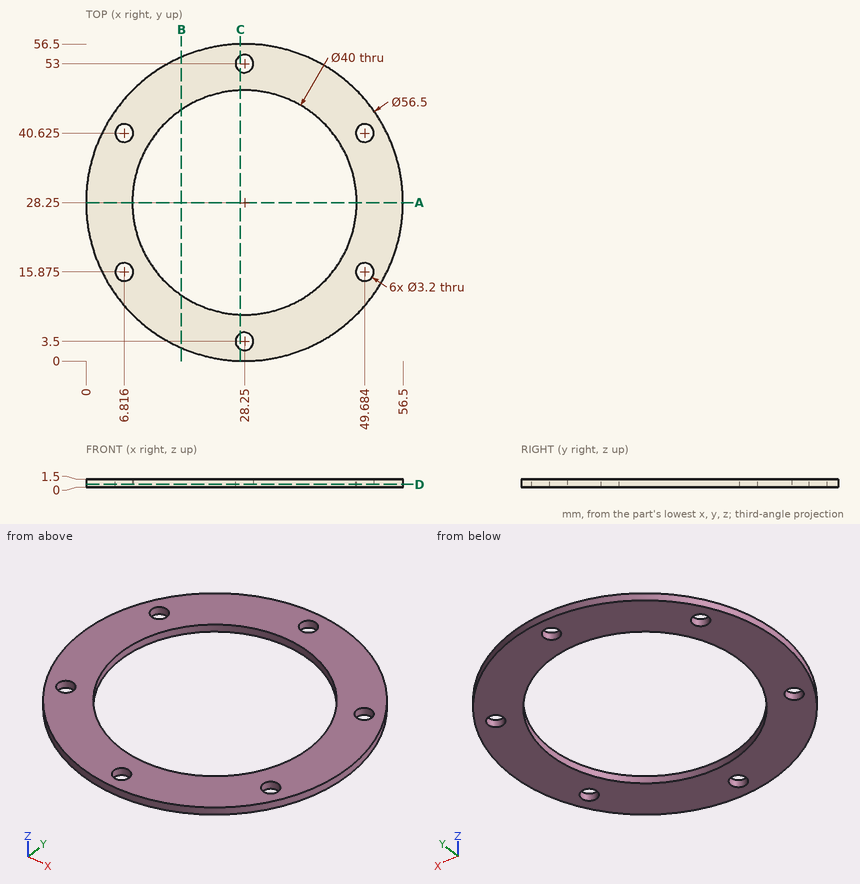
Job drawing, mm, ordinate dimensions from the low corner. One solid piece. Round coordinates to 2 decimals unless told otherwise and drop trailing zeros. Loops run counter-clockwise (first coordinate to the right, second up) from the corner with the lowest first, then second, coordinate; pieces in that order, holes last. Notation, with made-up numbers: (26, -6.75) -> (65, -6.75) arc R14 cw to (65, 12.25) -> close; hole circle Ø9 at (0, -4.5). An arc over 180 degrees is marked (long way). Use CSV: the item, a comma, the result in double quotes. Start each with the question number.
Q1. Saw through at C-C on x = 27.5. Give the cut face in (y, z).
Q2. Saw through at B-B on x = 17. Give the cut face in (y, z).
Q3. Drill centre lines: L1, parallel to Y at x = 28.25, z = 1.05; L2, parallel to X at y = 41, z = 0.45; L3, parallel to X at y = 17, z = 1. Where is each one in solid material? Low to high.
Q4. Saw through at A-A on y = 28.25. Give the cut face in (x, z).
Q5. Saw through at D-D on z = 0.55. Give the cut face in (x, y) (3 decimals).
Solutions:
1,outline,"(0.01, 0) -> (2.09, 0) -> (2.09, 1.5) -> (0.01, 1.5) -> close; (4.91, 0) -> (8.26, 0) -> (8.26, 1.5) -> (4.91, 1.5) -> close; (48.24, 0) -> (51.59, 0) -> (51.59, 1.5) -> (48.24, 1.5) -> close; (54.41, 0) -> (56.49, 0) -> (56.49, 1.5) -> (54.41, 1.5) -> close"
2,outline,"(2.34, 0) -> (11.71, 0) -> (11.71, 1.5) -> (2.34, 1.5) -> close; (44.79, 0) -> (54.16, 0) -> (54.16, 1.5) -> (44.79, 1.5) -> close"
3,L1,"y = 0 to 1.9, 5.1 to 8.25, 48.25 to 51.4, 54.6 to 56.5"
3,L2,"x = 3.04 to 5.26, 8.37 to 12.84, 43.66 to 48.13, 51.24 to 53.46"
3,L3,"x = 2.34 to 5.68, 7.95 to 11.71, 44.79 to 48.55, 50.82 to 54.16"
4,outline,"(0, 0) -> (8.25, 0) -> (8.25, 1.5) -> (0, 1.5) -> close; (48.25, 0) -> (56.5, 0) -> (56.5, 1.5) -> (48.25, 1.5) -> close"
5,outline,"circle Ø56.5 at (28.25, 28.25); hole circle Ø3.2 at (6.816, 15.875); hole circle Ø3.2 at (6.816, 40.625); hole circle Ø40 at (28.25, 28.25); hole circle Ø3.2 at (28.25, 3.5); hole circle Ø3.2 at (28.25, 53); hole circle Ø3.2 at (49.684, 15.875); hole circle Ø3.2 at (49.684, 40.625)"
